```python
from build123d import *

# Parameters (mm, degrees)
F0_R     = 16.25
F1_DEPTH = 3
F2_R     = 15.4
F3_DEPTH = 3.001
F4_SIZE  = 0.8


with BuildPart() as f1:
    # F0 (on Top) → F1 (new body)
    with BuildSketch(Plane.XY):
        Circle(F0_R)
    extrude(amount=F1_DEPTH)

    # F2 (on face) → F3 (cut, through all)
    with BuildSketch(Plane.XY.offset(3)):
        Circle(F2_R)
    extrude(amount=-F3_DEPTH, mode=Mode.SUBTRACT)

    # F4
    f4_edges = [f1.edges().sort_by_distance(p)[0] for p in [
        (-15.4, 0, 3),
        (-15.4, 0, 0),
    ]]
    chamfer(f4_edges, length=F4_SIZE)


solid = f1.part
```
Can you work these out from the model? Positions are in its coordinate system, mm. Coordinates: 2 decimals unless noted, no trailing zeros. Loops run counter-clockwise (first coordinate to the right, second up) from the corner with the lowest first, then second, coordinate; pieces in that order, holes last. Notation, with made-up numbers: M -21,47 L -17,47 A15 ccw -17,52 Z; hole C -4.75,-25.5 d7. An arc over 180 degrees is marked long. Put each result on its own line as item: value. Start each with the question number.
(1) Imagine slicing it at A-A on y = 0. List the corners of the cut face in (x, z) for me.
(2) We'd pull the mould along X, two halves only. Please class faces 1 (the face through (-3.338, -15.034, 1.51)), 2 (the face through (15.5, 4.88, 1.48)): +X half, -X half, draft (parallel to the pull), parting line (faces both ways), or undercut.
(3) Will this pin go through, and if not, where does the flat tip stop? pin 1 Ø18.5 at (x, y) = (0, 0) entering from -Z.
(4) I need wall thicknesses on probe 1 along Y at (x, z) = (0, 1.4); probe 2 along X at (y, z) = (-8.5, 0.3); probe 3 along Y at (x, z) = (-7, 2.6) (3 decimals). Which ranges of each line are inside material? Lowest first, please.
(5) Imagine slicing it at C-C on z = 1.35. List the corners of the cut face in (x, y) for me.
Worked answers:
1. outline: M -16.25,0 L -16.2,0 L -15.4,0.8 L -15.4,2.2 L -16.2,3 L -16.25,3 Z; M 15.4,0.8 L 16.2,0 L 16.25,0 L 16.25,3 L 16.2,3 L 15.4,2.2 Z
2. face 1: undercut
2. face 2: parting line
3. pin 1: passes through
4. probe 1: y = -16.25 to -15.4, 15.4 to 16.25
4. probe 2: x = -13.85 to -13.44, 13.44 to 13.85
4. probe 3: y = -14.665 to -14.165, 14.165 to 14.665
5. outline: C 0,0 d32.5; hole C 0,0 d30.8
